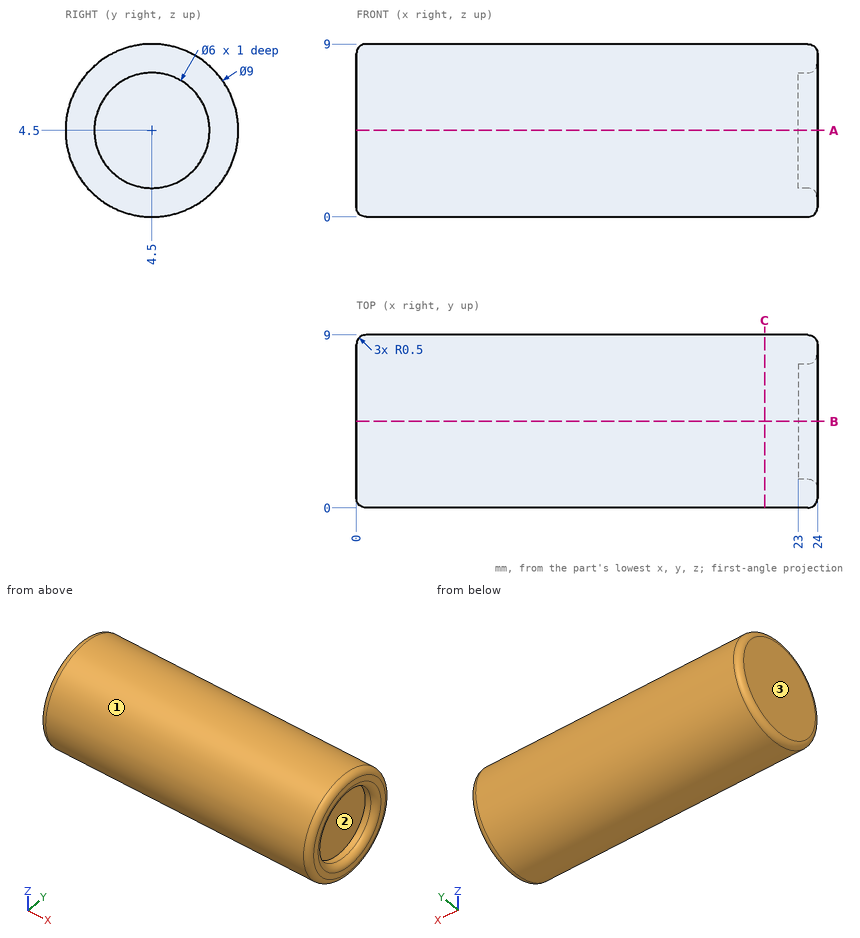
Check sheet for the drawn part. Datum: minimum x, y, z corner. Units: mm. Round coordinates to 2 decimals unless told otherwise and drop trailing zeros. Loops run counter-clockwise (first coordinate to the right, second up) from the corner with the lowest first, then second, coordinate; pieces in that order, holes last. Notation, with made-up numbers: (15, 86.25) - (50, 86.25) arc R18 cw to (50, 112.25) - close; hole circle Ø11 at (-9.75, 88.5). An arc over 180 degrees is marked (long way). Write item = value, one per line. Start each with the question number.
1. Section check C-C on x = 21.25. Enter the section's corners in (y, z), then the cut area to 3 significant figures.
2. Mould release check, pull along Z, two halves, no side actions. Record for the marked faces 1, 2 and 3: released by +Z, released by -Z, zero draft, split by the parting line, or undercut.
3. Depth check by flat-ended pin: pin 1 (2 mm diameter, centred on x = 10, z = 6, fed in from +Y); pin 2 (1.8 mm diameter, centred on y = 3.5, z = 4, fed in from +X); pin 3 (3 mm diameter, centred on x = 4, y = 7, fed in from +Z). Enter the tip coordinate at first touch or a pass-through.
4. Section check A-A on z = 4.5. Enter the section's corners in (x, y).
5. Thickness scan on line 1 (Y direction, x = 23.35, z = 4.5); line 2 (X direction, y = 2.25, z = 3.75); line 3 (X direction, y = 0.75, z = 6). Record the ranges inside material, lowest first.
Working result:
q1.outline = circle Ø9 at (4.5, 4.5)
q1.area = 63.6 mm^2
q2.face_1 = split by the parting line
q2.face_2 = undercut
q2.face_3 = zero draft
q3.pin_1 = 8.97
q3.pin_2 = 23
q3.pin_3 = 8.89
q4.outline = (0, 0.5) arc R0.5 ccw to (0.5, 0) - (23.5, 0) arc R0.5 ccw to (24, 0.5) - (24, 1) arc R0.5 ccw to (23.5, 1.5) - (23, 1.5) - (23, 7.5) - (23.5, 7.5) arc R0.5 ccw to (24, 8) - (24, 8.5) arc R0.5 ccw to (23.5, 9) - (0.5, 9) arc R0.5 ccw to (0, 8.5) - close
q5.line_1 = 0 to 1.5, 7.5 to 9
q5.line_2 = 0 to 23
q5.line_3 = 0 to 24
